Here's how the part is built. I have some questions about the finished solid (model axes, mm). A direction names the side the tool comes from. Round coordinates to 2 decimals unless told otherwise and drop trailing zeros. Write each loop counter-clockwise with the first axis right and the second up, starting at its lowest first coordinate (ties: lowest second). Pieces come first, ordered by that corner, then holes. Notation, with made-up numbers: (-19.75, 7) - (18.25, 7) arc R17 cw to (18.25, 24) - close; hole circle Ø2 at (71.25, 58.5). An arc over 180 degrees is marked (long way). One line per question, with ' | ' between items. Start each with the question number.
(1) Imagine slicing it at B-B (y = 52). Write out the boundary of the cut face in (x, z).
(2) Will these pins go through, and if not, where does the flat tip stop? pin 1 (1.5 mm diameter, centred on x = 37, z = 4, fed in from +Y); pin 2 (12 mm diameter, centred on x = 130.5, y = 43, fed in from -Z); pin 3 (2.5 mm diameter, centred on y = 0.5, z = 22, fed in from +X).
(3) For faces 1 (the flat face through (25.4, 0, 23)), 2 (the flat face through (75, 2.54, 17)), 3 (the flat face through (127, 0, -5)), 4 (the flat face through (76, 0, 9)), which set-ups out of +Z, -Z, +X, -X, +Y, -Y let a thin tool reach every point of the face, with its end or its side?
(4) Imagine slicing it at C-C (z = -5.08). Write out the boundary of the cut face in (x, y), plus the area to 3 significant figures.
(5) Thinking about a two-plate mould opening in X: for faces 5 (the flat face through (20, 0, 27.94)), 6 (the cylindrical face through (129.923, 0.036, 22.765)), 7 (the flat face through (137.16, 0, -5)), which applies, pulls with the +X half, pulls with the -X half, needs draft (parallel to the pull), parting line crosses it, or undercut?
(6) If I drill on L1, parallel to Z at x = 20, y = -1; L2, parallel to Z at x = 20, y = 1; L3, parallel to X at y = 8, z = 5.5, over which ranges is the centre line in solid material (lowest first)?
(7) Imagine slicing it at D-D (x = 98). Write out the boundary of the cut face in (y, z), plus the area to 3 significant figures.
(8) Imagine slicing it at A-A (x = 132.08). Write out the boundary of the cut face in (y, z).
Autodesk Inventor part; units mm, degrees
ref_plane "YZ Plane" through (0, 0, 0) normal (1, 0, 0) x (0, 1, 0)
ref_plane "XZ Plane" through (0, 0, 0) normal (0, 1, 0) x (-1, 0, 0)
ref_plane "XY Plane" through (0, 0, 0) normal (0, 0, 1) x (1, 0, 0)
sketch "Sketch1" plane through (0, 0, 0) normal (0, 0, 1) x (1, 0, 0)
  line L0 (0, 0) -> (0, 67.31)
  line L1 (0, 67.31) -> (149.86, 67.31)
  line L2 (149.86, 67.31) -> (149.86, 0)
  line L3 (149.86, 0) -> (0, 0)
  line L4 (-2.54, 69.85) -> (-2.54, -2.54)
  line L5 (-2.54, -2.54) -> (152.4, -2.54)
  line L6 (152.4, -2.54) -> (152.4, 69.85)
  line L7 (152.4, 69.85) -> (-2.54, 69.85)
  dimension "d0" = 67.31
  dimension "d1" = 149.86
  dimension "d5" = 72.39
  dimension "d6" = 154.94
  dimension "d7" = 72.39
extrude "Extrusion1" add sketch "Sketch1" along normal blind 17.78
sketch "Sketch2" plane through (0, 0, 0) normal (1, 0, 0) x (0, 0, -1)
  line L0 (0, 0) -> (-2.54, 0)
  line L1 (0, 0) -> (-17.78, 0)
  line L2 (-2.54, 0) -> (-2.54, 67.31)
  line L3 (0, 67.31) -> (-17.78, 67.31)
  line L4 (-2.54, 67.31) -> (0, 67.31)
  line L5 (0, 67.31) -> (0, 0)
  line L6 (0, 67.31) -> (0, 0)
  dimension "d10" = 2.54
extrude "Extrusion2" add sketch "Sketch2" along normal blind 2.54
sketch "Sketch3" plane through (0, 0, 17.78) normal (0, 1, 0) x (1, 0, 0)
  line L0 (0, 15.24) -> (0, 0)
  line L1 (0, 2.54) -> (149.86, 2.54)
  line L2 (149.86, 2.54) -> (149.86, 0)
  line L3 (149.86, 0) -> (0, 0)
  line L4 (0, 0) -> (149.86, 0)
  point P0 (0, 17.78)
extrude "Extrusion3" add sketch "Sketch3" along normal blind 2.54
sketch "Sketch4" plane through (-2.54, 69.85, 0) normal (0, 1, 0) x (1, 0, 0)
  line L0 (2.54, -15.24) -> (2.54, -2.54)
  line L1 (2.54, -2.54) -> (2.54, -15.24)
  line L2 (2.54, -2.54) -> (152.4, -2.54)
  line L3 (152.4, 0) -> (152.4, -15.24)
  line L4 (152.4, -15.24) -> (2.54, -15.24)
  point P0 (2.54, 0)
extrude "Extrusion4" cut sketch "Sketch4" against normal blind 2.54
sketch "Sketch5" plane through (0, 67.31, 17.78) normal (0, -1, 0) x (1, 0, 0)
  line L0 (149.86, 0) -> (149.86, -2.54)
  line L1 (149.86, -2.54) -> (0, -2.54)
  line L2 (0, -2.54) -> (0, 0)
  line L3 (0, 0) -> (149.86, 0)
  point P0 (0, -17.78)
extrude "Extrusion5" add sketch "Sketch5" along normal blind 2.54
sketch "Sketch6" plane through (0, 0, 2.54) normal (1, 0, 0) x (0, 0, -1)
  line L0 (-12.7, 2.54) -> (-15.24, 2.54)
  line L1 (-15.24, 2.54) -> (-15.24, 64.77)
  line L2 (-15.24, -2.54) -> (-15.24, 69.85)
  line L3 (-15.24, 64.77) -> (-12.7, 64.77)
  line L4 (-12.7, 64.77) -> (-12.7, 2.54)
  point P0 (2.54, 0)
  dimension "d19" = 62.23
extrude "Extrusion6" add sketch "Sketch6" along normal blind 2.54
sketch "Sketch7" plane through (0, 2.54, 17.78) normal (0, 1, 0) x (1, 0, 0)
  line L0 (149.86, 2.54) -> (149.86, 0)
  line L1 (149.86, 0) -> (147.32, 0)
  line L2 (149.86, 0) -> (2.54, 0)
  line L3 (147.32, 0) -> (147.32, 2.54)
  line L4 (147.32, 2.54) -> (149.86, 2.54)
  point P0 (0, 17.78)
  dimension "d22" = 2.54
extrude "Extrusion7" add sketch "Sketch7" along normal blind 62.23
sketch "Sketch8" plane through (149.86, 0, 0) normal (-1, 0, 0) x (0, 0, 1)
  line L0 (0, 0) -> (2.54, 0)
  line L1 (2.54, 0) -> (2.54, 2.54)
  line L2 (2.54, 69.85) -> (2.54, 0)
  line L3 (2.54, 2.54) -> (0, 2.54)
  line L4 (0, 0) -> (0, 67.31)
  dimension "d25" = 2.54
extrude "Extrusion8" add sketch "Sketch8" along normal blind 149.86
sketch "Sketch9" plane through (149.86, 67.31, 2.54) normal (-1, 0, 0) x (0, 0, 1)
  line L0 (-2.54, 0) -> (0, 0)
  line L1 (0, 0) -> (0, -2.54)
  line L2 (0, 0) -> (0, -64.77)
  line L3 (0, -2.54) -> (-2.54, -2.54)
  line L4 (-2.54, -64.77) -> (-2.54, 0)
  point P0 (-2.54, -67.31)
  point P1 (0, -67.31)
  dimension "d28" = 2.54
  dimension "d29" = 2.54
extrude "Extrusion9" add sketch "Sketch9" along normal blind 149.86
sketch "Sketch10" plane through (149.86, 0, 15.24) normal (-1, 0, 0) x (0, 0, 1)
  line L0 (-15.24, 2.54) -> (-12.7, 2.54)
  line L1 (-12.7, 2.54) -> (-12.7, 64.77)
  line L2 (-12.7, 64.77) -> (-15.24, 64.77)
  line L3 (-15.24, -2.54) -> (-15.24, 69.85)
  point P0 (-15.24, 0)
extrude "Extrusion10" add sketch "Sketch10" along normal blind 74.93
sketch "Sketch11" plane through (0, 0, 17.78) normal (0, 0, 1) x (1, 0, 0)
  line L0 (147.32, 2.54) -> (2.54, 2.54)
  line L1 (15.24, 2.54) -> (15.24, -2.54)
  line L2 (-2.54, -2.54) -> (152.4, -2.54)
  line L3 (15.24, -2.54) -> (25.4, -2.54)
  line L4 (25.4, -2.54) -> (25.4, 2.54)
  point P0 (0, 0)
  dimension "d34" = 10.16
extrude "Extrusion11" add sketch "Sketch11" along normal blind 10.16
sketch "Sketch12" plane through (0, 2.54, 17.78) normal (0, 1, 0) x (1, 0, 0)
  line L0 (15.24, 0) -> (15.24, -5.08)
  line L1 (15.24, 0) -> (15.24, -10.16)
  line L2 (15.24, -5.08) -> (20.32, -5.08)
  circle A0 centre (20.32, -5.08) radius 2.159
  point P0 (0, 17.78)
  dimension "d37" = 5.08
  dimension "d38" = 5.08
  dimension "d39" = 4.318
extrude "Extrusion12" cut sketch "Sketch12" against normal blind 10.16
sketch "Sketch13" plane through (0, 0, 17.78) normal (0, 0, 1) x (1, 0, 0)
  line L0 (149.86, 0) -> (137.16, 0)
  line L1 (0, 0) -> (149.86, 0)
  line L2 (137.16, 0) -> (137.16, 2.54)
  line L3 (147.32, 2.54) -> (2.54, 2.54)
  line L4 (137.16, 2.54) -> (127, 2.54)
  line L5 (127, 2.54) -> (127, -2.54)
  line L6 (25.4, -2.54) -> (152.4, -2.54)
  line L7 (137.16, -2.54) -> (137.16, 0)
  dimension "d42" = 12.7
  dimension "d43" = 10.16
extrude "Extrusion13" add sketch "Sketch13" along normal blind 10.16
sketch "Sketch14" plane through (0, 2.54, 17.78) normal (0, 1, 0) x (1, 0, 0)
  line L0 (127, 0) -> (127, -5.08)
  line L1 (127, 0) -> (127, -10.16)
  line L2 (127, -5.08) -> (132.08, -5.08)
  circle A0 centre (132.08, -5.08) radius 2.159
  point P0 (0, 17.78)
  dimension "d46" = 5.08
  dimension "d47" = 5.08
  dimension "d48" = 4.318
extrude "Extrusion14" cut sketch "Sketch14" against normal blind 10.16
sketch "Sketch15" plane through (0, 0, 0) normal (0, 0, -1) x (-1, 0, 0)
  line L0 (0, 0) -> (-149.86, 0)
  line L1 (-15.24, 0) -> (-15.24, 2.54)
  line L2 (-74.93, 2.54) -> (-2.54, 2.54)
  line L3 (-15.24, 2.54) -> (-25.4, 2.54)
  line L4 (-25.4, 2.54) -> (-25.4, -2.54)
  line L5 (-15.24, -2.54) -> (-25.4, -2.54)
  line L6 (-25.4, -2.54) -> (-15.24, -2.54)
  line L7 (-15.24, -2.54) -> (-15.24, 2.54)
  dimension "d51" = 10.16
extrude "Extrusion15" add sketch "Sketch15" along normal blind 10.16
sketch "Sketch16" plane through (2.54, 2.54, 2.54) normal (0, 1, 0) x (1, 0, 0)
  line L0 (12.7, 2.54) -> (12.7, 7.62)
  line L1 (12.7, 2.54) -> (12.7, 12.7)
  line L2 (12.7, 7.62) -> (17.78, 7.62)
  circle A0 centre (17.78, 7.62) radius 2.159
  point P0 (-2.54, 2.54)
  dimension "d54" = 5.08
  dimension "d55" = 5.08
  dimension "d56" = 4.318
extrude "Extrusion16" cut sketch "Sketch16" against normal blind 10.16
sketch "Sketch17" plane through (0, 0, 0) normal (0, 0, -1) x (-1, 0, 0)
  line L0 (-149.86, 69.85) -> (-149.86, 0)
  line L1 (-149.86, 2.54) -> (-137.16, 2.54)
  line L2 (-137.16, 2.54) -> (-147.32, 2.54)
  line L3 (-137.16, 2.54) -> (-137.16, -2.54)
  line L4 (0, 0) -> (-149.86, 0)
  line L5 (-137.16, -2.54) -> (-127, -2.54)
  line L6 (-127, -2.54) -> (-137.16, -2.54)
  line L7 (-127, -2.54) -> (-127, 2.54)
  line L8 (-127, 2.54) -> (-137.16, 2.54)
  line L9 (-137.16, 2.54) -> (-127, 2.54)
  dimension "d59" = 12.7
  dimension "d60" = 10.16
extrude "Extrusion17" add sketch "Sketch17" along normal blind 10.16 contours L4 L7 L5 L3 | L3 L8 L7 L4
sketch "Sketch18" plane through (127, 2.54, 0) normal (0, 1, 0) x (1, 0, 0)
  line L0 (0, 0) -> (0, 5.08)
  line L1 (0, 0) -> (0, 10.16)
  line L2 (0, 5.08) -> (5.08, 5.08)
  circle A0 centre (5.08, 5.08) radius 2.159
  point P0 (-127, 0)
  dimension "d63" = 5.08
  dimension "d64" = 5.08
  dimension "d65" = 4.318
extrude "Extrusion18" cut sketch "Sketch18" against normal blind 10.16
properties part number "PhoneCase"
Check sheet entries:
1) outline: (-2.54, 0) - (2.54, 0) - (2.54, 2.54) - (0, 2.54) - (0, 15.24) - (2.54, 15.24) - (2.54, 17.78) - (-2.54, 17.78) - close; (74.93, 0) - (152.4, 0) - (152.4, 17.78) - (147.32, 17.78) - (147.32, 15.24) - (149.86, 15.24) - (149.86, 2.54) - (74.93, 2.54) - close
2) pin 1: y = 0 | pin 2: z = 0 | pin 3: x = 137.16
3) face 1: +Z, +Y, -Y | face 2: +Z | face 3: -Z, +Y, -Y | face 4: +Y
4) outline: (15.24, -2.54) - (18.16, -2.54) - (18.16, 2.54) - (15.24, 2.54) - close; (22.48, -2.54) - (25.4, -2.54) - (25.4, 2.54) - (22.48, 2.54) - close; (127, -2.54) - (129.92, -2.54) - (129.92, 2.54) - (127, 2.54) - close; (134.24, -2.54) - (137.16, -2.54) - (137.16, 2.54) - (134.24, 2.54) - close | area: 59.4 mm^2
5) face 5: needs draft | face 6: undercut | face 7: pulls with the +X half
6) L1: -10.16 to -7.22, -2.94 to 20.72, 25 to 27.94 | L2: -10.16 to -7.22, -2.94 to 2.54, 15.24 to 20.72, 25 to 27.94 | L3: -2.54 to 0, 149.86 to 152.4
7) outline: (-2.54, 0) - (69.85, 0) - (69.85, 2.54) - (0, 2.54) - (0, 15.24) - (2.54, 15.24) - (2.54, 17.78) - (-2.54, 17.78) - close; (64.77, 15.24) - (69.85, 15.24) - (69.85, 17.78) - (64.77, 17.78) - close | area: 242 mm^2
8) outline: (-2.54, -10.16) - (2.54, -10.16) - (2.54, -7.24) - (-2.54, -7.24) - close; (-2.54, -2.92) - (2.54, -2.92) - (2.54, 0) - (69.85, 0) - (69.85, 2.54) - (0, 2.54) - (0, 15.24) - (2.54, 15.24) - (2.54, 20.7) - (-2.54, 20.7) - close; (-2.54, 25.02) - (2.54, 25.02) - (2.54, 27.94) - (-2.54, 27.94) - close; (64.77, 15.24) - (69.85, 15.24) - (69.85, 17.78) - (64.77, 17.78) - close
